The model under review builds one solid part; all positions refer to its coordinate system, in mm. A direction names the side the tool comes from. Round coordinates to 2 decimals unless told otherwise and drop trailing zeros. Loops run counter-clockwise (first coordinate to the right, second up) from the corner with the lowest first, then second, coordinate; pieces in that order, holes last. Notation, with made-up numbers: M -14.5,53 L 30.5,53 A10 ccw 30.5,64 Z; hole C 82,81 d4. An arc over 180 degrees is marked long. One line per question, with ' | ' between items.
from build123d import *

# Parameters (mm, degrees)
F0_R     = 65.653688
F0_R_2   = 38.1
F1_DEPTH = 50.546
F0_R_3   = 25.4
F2_DEPTH = 19.558
F3_SIZE  = 12.7


with BuildPart() as f1:
    # F0 (on Top) → F1 (new body)
    with BuildSketch(Plane.XY):
        Circle(F0_R)
        Circle(F0_R_2, mode=Mode.SUBTRACT)
    extrude(amount=F1_DEPTH)

    # F0 (on Top) → F2 (join)
    with BuildSketch(Plane.XY):
        Circle(F0_R_2)
        Circle(F0_R_3, mode=Mode.SUBTRACT)
    extrude(amount=F2_DEPTH)

    # F3
    f3_edges = [f1.edges().sort_by_distance(p)[0] for p in [
        (-25.4, 0, 0),
    ]]
    chamfer(f3_edges, length=F3_SIZE)


solid = f1.part
1) Mouldability with a two-part tool opening along Y and no side actions: class faces 1 (the cylindrical face through (62.622, 19.721, 24.919)), 2 (the cylindrical face through (-5.506, -24.796, 16.081)), 3 (the flat face through (28, -28, 50.546)) as +Y half, -Y half, draft (parallel to the pull), parting line (faces both ways), or undercut.
Output values:
face 1: parting line | face 2: undercut | face 3: draft
2) Insertion check: P1, Ø8, axis at y = 52, z = 34.5, coming from the -X side; P2, Ø2, axis at y = 34.5, z = 20.5, coming from the +X side; P3, Ø1, axis at x = -44, y = 16.5, coming from the -Z side; P4, Ø10, axis at x = -26.5, z = 14.5, coming from the +Y side. Each pin has a flat end and moves straight along its axis. Give the tip position at first contact, or say it passes through.
Output values:
P1: stops at x = -44.79 | P2: stops at x = 56.46 | P3: stops at z = 0 | P4: stops at y = 62.03
3) Add section C-C on z = 44.5. State the section outline as (x, y) points, then the cut area to 3 significant figures.
Output values:
outline: C 0,0 d131.31; hole C 0,0 d76.2 | area: 8,980 mm²
4) For line 1 (Y direction, x = 0.5, z = 34.5); line 2 (Y direction, x = 0, z = 16); line 3 (X direction, y = 27.5, z = 20), list the stretches that pass through material, from the lowest coordinate up.
Output values:
line 1: y = -65.65 to -38.1, 38.1 to 65.65 | line 2: y = -65.65 to -25.4, 25.4 to 65.65 | line 3: x = -59.62 to -26.37, 26.37 to 59.62
5) Add section D-D on x = -50.5. State the section outline as (y, z) points.
Output values:
outline: M -41.95,0 L 41.95,0 L 41.95,50.55 L -41.95,50.55 Z
6) Machinability: for faces 4 (the flat face through (28, -28, 0)), 5 (the cylindrical face through (-30.235, -23.183, 34.835)), which of the approach directions +Z, -Z, +X, -X, +Y, -Y give a long, thin tool a straight path to every point of the face, cutting with its end or side? Answer none if there is none.
Output values:
face 4: -Z, +X, -X, +Y, -Y | face 5: +Z
7) Add section A-A on x = 0. State the section outline as (y, z) points.
Output values:
outline: M -65.65,0 L -38.1,0 L -25.4,12.7 L -25.4,19.56 L -38.1,19.56 L -38.1,50.55 L -65.65,50.55 Z; M 25.4,12.7 L 38.1,0 L 65.65,0 L 65.65,50.55 L 38.1,50.55 L 38.1,19.56 L 25.4,19.56 Z
